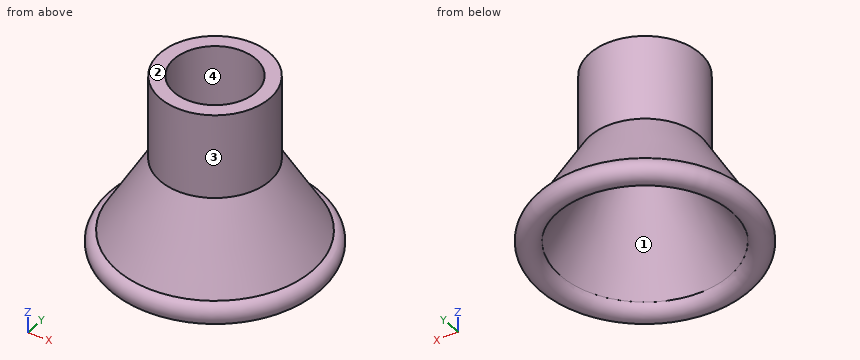
from build123d import *


# Not quite as in the source:
# - a feature names something its author has since deleted; it is built from what else it names


with BuildPart() as f1:
    # F0 (on Front) → F1 (revolve)
    with BuildSketch(Plane.XZ):
        with BuildLine():
            Line((9.2075, 19.05), (9.2075, 2.54))
            Line((9.2075, 2.54), (7.9375, 2.54))
            Line((7.9375, 2.54), (7.9375, 0))
            Line((7.9375, 0), (19.05, -19.05))
            ThreePointArc((19.05, -19.05), (23.2206068806, -20.9974910015), (22.0363946464, -16.5495336796))
            Line((22.0363946464, -16.5495336796), (12.3825, 0))
            Line((12.3825, 0), (12.3825, 19.05))
            Line((12.3825, 19.05), (9.2075, 19.05))
        make_face()
    revolve(axis=Axis((0, 0, -5.8383159339), (0, 0, -1)))


solid = f1.part
Verification items for the finished model (mm, model axes). Face numbers are marked on the shaded views. Give positions to 0.01 mm unless a question says otherwise; leave off trailing zeros. Loops run counter-clockwise (first coordinate to the right, second up) from the corner with the lowest first, then second, coordinate; pieces in that order, holes last.
1. Cross-section at C-C on z = 13.5. Record the cut outline in (x, y) (1 decimal), and give its area (3 significant figures).
Derived:
outline: circle Ø24.8 at (0, 0); hole circle Ø18.4 at (0, 0)
area: 215 mm2
2. Cross-section at D-D on z = -15.5. Record the cut outline in (x, y).
Derived:
outline: circle Ø42.85 at (0, 0); hole circle Ø33.96 at (0, 0)
3. Release check for a two-part mould opening along X. For the marked faces 1, 2, 3 and 4 record: +X half, -X half, draft (parallel to the pull), parting line (faces both ways), or undercut.
Derived:
face 1: undercut
face 2: draft
face 3: parting line
face 4: undercut
4. Go/stop test with flat-tipped pins: P1, Ø8, axis at x = 4.5, y = -19, coming from the +Z side; P2, Ø10, axis at y = 14.5, z = 1, coming from the -X side; P3, Ø3, axis at x = 10.5, y = -17.5, coming from the -Z side; P4, Ø4, axis at x = 6.5, z = 5.5, coming from the +Y side. Record where each tip stops, or that it passes through.
Derived:
P1: stops at z = -5.39
P2: stops at x = -8.56
P3: stops at z = -21.59
P4: stops at y = 11.54
5. Material ranges on probe 1 along X at (y, z) = (0, 11); probe 2 along X at (y, z) = (0, 1); probe 3 along Y at (x, z) = (8, 12.5), recorded low to high.
Derived:
probe 1: x = -12.38 to -9.21, 9.21 to 12.38
probe 2: x = -12.38 to -7.94, 7.94 to 12.38
probe 3: y = -9.45 to -4.56, 4.56 to 9.45
6. Cross-section at A-A on x = 0. Record the cut outline in (y, z).
Derived:
outline: (-22.04, -16.55) arc R2.54 ccw (long way) to (-19.05, -19.05) - (-7.94, 0) - (-7.94, 2.54) - (-9.21, 2.54) - (-9.21, 19.05) - (-12.38, 19.05) - (-12.38, 0) - close; (7.94, 0) - (19.05, -19.05) arc R2.54 ccw (long way) to (22.04, -16.55) - (12.38, 0) - (12.38, 19.05) - (9.21, 19.05) - (9.21, 2.54) - (7.94, 2.54) - close
